```python
from build123d import *

# Parameters (mm, degrees)
SKETCH1_W           = 40.5
SKETCH1_H           = 20
BOSS_EXTRUDE1_DEPTH = 41
SKETCH2_W           = 56.4
SKETCH2_H           = 20
SKETCH2_R           = 2.25
BOSS_EXTRUDE2_DEPTH = 3.5
SKETCH3_R           = 3
BOSS_EXTRUDE3_DEPTH = 6
SKETCH4_W           = 10
SKETCH4_H           = 3.5
BOSS_EXTRUDE4_DEPTH = 5
FILLET1_R           = 2
FILLET2_R           = 1
FILLET3_R           = 1
SKETCH5_R           = 9.75
BOSS_EXTRUDE5_DEPTH = 2
SKETCH6_R           = 7
SKETCH6_R_2         = 4
BOSS_EXTRUDE6_DEPTH = 4


with BuildPart() as part:
    # Sketch1 → Boss-Extrude1 (new body)
    with BuildSketch(Plane(origin=(0, 0, 0), x_dir=(1, 0, 0), z_dir=(0, 1, 0))):
        Rectangle(SKETCH1_W, SKETCH1_H)
    extrude(amount=BOSS_EXTRUDE1_DEPTH)

    # Sketch2 → Boss-Extrude2 (add)
    with BuildSketch(Plane(origin=(0, 28, 0), x_dir=(-1, 0, 0), z_dir=(0, -1, 0))):
        Rectangle(SKETCH2_W, SKETCH2_H)
        with Locations(Location((-24, 5, 0), (0, 0, 90))):
            Circle(SKETCH2_R, mode=Mode.SUBTRACT)
        with Locations(Location((24, 5, 0), (0, 0, 90))):
            Circle(SKETCH2_R, mode=Mode.SUBTRACT)
        with Locations(Location((24, -5, 0), (0, 0, 90))):
            Circle(SKETCH2_R, mode=Mode.SUBTRACT)
        with Locations(Location((-24, -5, 0), (0, 0, 90))):
            Circle(SKETCH2_R, mode=Mode.SUBTRACT)
    extrude(amount=-BOSS_EXTRUDE2_DEPTH)

    # Sketch3 → Boss-Extrude3 (add)
    with BuildSketch(Plane(origin=(0, 41, 0), x_dir=(1, 0, 0), z_dir=(0, 1, 0))):
        with Locations(Location((-10.5, 0, 0), (0, 0, 270))):
            Circle(SKETCH3_R)
    extrude(amount=BOSS_EXTRUDE3_DEPTH)

    # Sketch4 → Boss-Extrude4 (add)
    with BuildSketch(Plane.ZY.offset(20.25)):
        with Locations((0, 5.25)):
            Rectangle(SKETCH4_W, SKETCH4_H)
    extrude(amount=BOSS_EXTRUDE4_DEPTH)

    # Fillet1
    fillet1_edges = [part.edges().sort_by_distance(p)[0] for p in [
        (28.2, 29.75, -10),
        (-28.2, 29.75, 10),
        (28.2, 29.75, 10),
        (-28.2, 29.75, -10),
    ]]
    fillet(fillet1_edges, radius=FILLET1_R)

    # Fillet2
    fillet2_edges = [part.edges().sort_by_distance(p)[0] for p in [
        (20.25, 14, 10),
        (-20.25, 14, 10),
        (-20.25, 14, -10),
        (20.25, 14, -10),
        (0, 0, 10),
        (-20.25, 0, 0),
        (0, 0, -10),
        (20.25, 0, 0),
        (-20.25, 36.25, 10),
        (-20.25, 36.25, -10),
    ]]
    fillet(fillet2_edges, radius=FILLET2_R)

    # Fillet3
    fillet3_edges = [part.edges().sort_by_distance(p)[0] for p in [
        (0.5, 41, 10),
        (-20.25, 41, 0),
        (-19.957106781, 41, 9.707106781),
        (-19.957106781, 41, -9.707106781),
        (20.25, 41, 0),
        (20.25, 36.25, 10),
        (20.25, 36.25, -10),
        (0.5, 41, -10),
    ]]
    fillet(fillet3_edges, radius=FILLET3_R)

    # Sketch5 → Boss-Extrude5 (add)
    with BuildSketch(Plane(origin=(0, 47, 0), x_dir=(1, 0, 0), z_dir=(0, 1, 0))):
        with Locations(Location((-10.5, 0, 0), (0, 0, 270))):
            Circle(SKETCH5_R)
    extrude(amount=BOSS_EXTRUDE5_DEPTH)

    # Sketch6 → Boss-Extrude6 (add)
    with BuildSketch(Plane.XZ):
        with Locations(Location((-10.5, 0, 0), (0, 0, 90))):
            Circle(SKETCH6_R)
        with Locations(Location((-10.5, 0, 0), (0, 0, 270))):
            Circle(SKETCH6_R_2, mode=Mode.SUBTRACT)
    extrude(amount=BOSS_EXTRUDE6_DEPTH)


solid = part.part
```
The model under review builds one solid part; all positions refer to its coordinate system, in mm. A direction names the side the tool comes from. Round coordinates to 2 decimals unless told otherwise and drop trailing zeros. Loops run counter-clockwise (first coordinate to the right, second up) from the corner with the lowest first, then second, coordinate; pieces in that order, holes last. Notation, with made-up numbers: M -34,-25 L -4,-25 A11 ccw -4,-18 Z; hole C 27,7 d10. An arc over 180 degrees is marked long. Answer as a JSON object with one key per item and string values.
(1) Draft analysis for pull direction X (two halves, no side actions). For faces 6 (the cylindrical face through (-26.196, 29.726, 5.488)), 7 (the cylindrical face through (-7.526, 43.958, -0.391)), 8 (the flat face through (0, 20, -10)), state which applies: released by +X, released by -X, zero draft, split by the parting line, or undercut.
Resolved:
{"face 6": "undercut", "face 7": "split by the parting line", "face 8": "zero draft"}
(2) Take a section at C-C on y = 35. Give the boundary of the cut face in (x, z).
Resolved:
{"outline": "M -20.25,-9 A1 ccw -19.25,-10 L 19.25,-10 A1 ccw 20.25,-9 L 20.25,9 A1 ccw 19.25,10 L -19.25,10 A1 ccw -20.25,9 Z"}
(3) Clearance check with flat-ended pins moving along their axes: P1, Ø3, axis at x = -23, y = 4.5, coming from the -Z side; P2, Ø9, axis at y = 15.5, z = 3.5, coming from the -X side; P3, Ø1, axis at x = -21.5, y = 41.5, coming from the -Z side; P4, Ø2.5, axis at x = -8.5, z = -1, coming from the -Y side. State where each tip first meets the part, or that it passes through.
Resolved:
{"P1": "z = -5", "P2": "x = -20.25", "P3": "through", "P4": "y = 0"}
(4) Take a section at B-B on x = -10.5. Give the boundary of the cut face in (y, z), and give its area (3 significant figures).
Resolved:
{"outline": "M -4,-7 L 0,-7 L 0,-9 A1 ccw 1,-10 L 40,-10 A1 ccw 41,-9 L 41,-3 L 47,-3 L 47,-9.75 L 49,-9.75 L 49,9.75 L 47,9.75 L 47,3 L 41,3 L 41,9 A1 ccw 40,10 L 1,10 A1 ccw 0,9 L 0,7 L -4,7 L -4,4 L 0,4 L 0,-4 L -4,-4 Z", "area": "918 mm²"}
(5) Tool access review of faces 1 (the flat face through (20.25, 36, 0)), 2 (the flat face through (-23, 3.5, 0)), 3 (the cylindrical face through (-27.6, 29.77, -9.43)), 4 (the cylindrical face through (-3.666, -1.972, -1.517)), 5 (the cylindrical face through (-26.196, 29.726, -4.512)): name each direction out of +Z, -Z, +X, -X, +Y, -Y from which nothing blocks a thin tool from reaching the whole face with its end or side.
Resolved:
{"face 1": "+Z, -Z, +X, +Y", "face 2": "+Z, -Z, -X, -Y", "face 3": "-Z, -X, +Y, -Y", "face 4": "-Y", "face 5": "+Y"}
(6) Take a section at D-D on x = 14.5. Give the boundary of the cut face in (y, z).
Resolved:
{"outline": "M 0,-9 A1 ccw 1,-10 L 40,-10 A1 ccw 41,-9 L 41,9 A1 ccw 40,10 L 1,10 A1 ccw 0,9 Z"}
(7) Take a section at A-A on x = 24. Give the boundary of the cut face in (y, z).
Resolved:
{"outline": "M 28,-10 L 31.5,-10 L 31.5,-7.25 L 28,-7.25 Z; M 28,-2.75 L 31.5,-2.75 L 31.5,2.75 L 28,2.75 Z; M 28,7.25 L 31.5,7.25 L 31.5,10 L 28,10 Z"}
(8) To check wall thickness, follow line 1 along X through (y, z) = (29.75, -5); line 2 along Y through (x, z) = (-5, 0.75); line 3 along Y through (x, z) = (-7, 8.5). State the ranges of each line that lie inside material, in increasing order.
Resolved:
{"line 1": "-28.2 to -26.25, -21.75 to 21.75, 26.25 to 28.2", "line 2": "-4 to 41, 47 to 49", "line 3": "0 to 41, 47 to 49"}
